Drawing for the job (mm, zero at the part's lowest x, y, z). A direction names the side the tool comes from. Round coordinates to 2 decimals unless told otherwise and drop trailing zeros. Write each loop counter-clockwise with the first axis right and the second up, starting at its lowest first coordinate (ties: lowest second). Pieces come first, ordered by that corner, then holes.
Item 1: Band-saw the part on B-B, the plane x = 150. Write the cut outline in (y, z).
Item 2: 3-axis set-ups, long thin cutter, end or side, ignore diameter. For the marked faces 1 and 2: which of +Z, -Z, +X, -X, +Y, -Y reach the whole face in a straight line?
Item 3: Band-saw the part on C-C, the plane z = 9. Write the cut outline in (x, y), then the cut area to 3 significant figures.
Item 4: Wall check: probe 1 along Y at (x, z) = (150, 10); probe 2 along Y at (x, z) = (136, 15); probe 3 along X at (y, z) = (16.5, 15). Give the ranges that are in metal, low to high.
Item 5: Band-saw the part on D-D, the plane x = 113. Write the cut outline in (y, z), then the cut area to 3 significant figures.
Item 6: Drop flat-ended pins along their axis: pin 1 Ø6 at (y, z) = (22, 8) entering from +X; pin 2 Ø9 at (x, y) = (150, 58.09) entering from -Z. Give the stop position or say it passes through.
Item 7: Band-saw the part on A-A, the plane y = 10. Write the cut outline in (x, z).
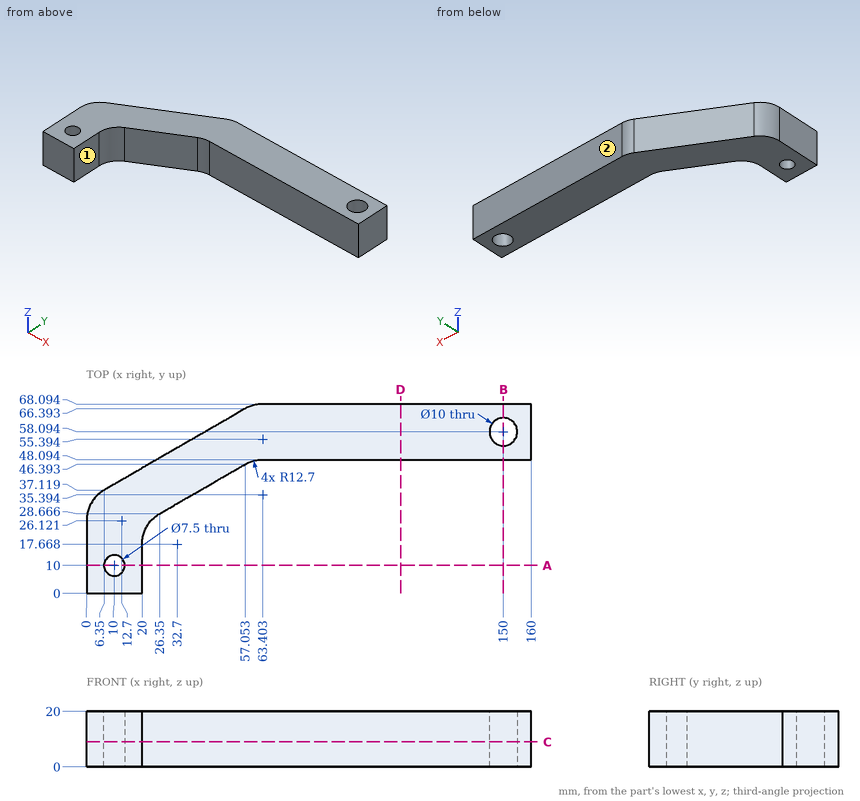
Results:
1. outline: (48.09, 0) - (53.09, 0) - (53.09, 20) - (48.09, 20) - close; (63.09, 0) - (68.09, 0) - (68.09, 20) - (63.09, 20) - close
2. face 1: +Z, -Z, +X, -Y
2. face 2: +Z, -Z, +X, -X, +Y
3. outline: (0, 0) - (20, 0) - (20, 17.67) arc R12.7 cw to (26.35, 28.67) - (57.05, 46.39) arc R12.7 cw to (63.4, 48.09) - (160, 48.09) - (160, 68.09) - (63.4, 68.09) arc R12.7 ccw to (57.05, 66.39) - (6.35, 37.12) arc R12.7 ccw to (0, 26.12) - close; hole circle Ø7.5 at (10, 10); hole circle Ø10 at (150, 58.09)
3. area: 3,460 mm2
4. probe 1: y = 48.09 to 53.09, 63.09 to 68.09
4. probe 2: y = 48.09 to 68.09
4. probe 3: x = 0 to 20
5. outline: (48.09, 0) - (68.09, 0) - (68.09, 20) - (48.09, 20) - close
5. area: 400 mm2
6. pin 1: stops at x = 22.33
6. pin 2: passes through
7. outline: (0, 0) - (6.25, 0) - (6.25, 20) - (0, 20) - close; (13.75, 0) - (20, 0) - (20, 20) - (13.75, 20) - close
